For this review, take the finished solid that the model builds, in its own axes (mm). Face numbers are marked on the shaded views. A direction names the side the tool comes from. Round coordinates to 2 decimals unless told otherwise and drop trailing zeros. Order: outer loops, then holes, each group sorted by start corner. A loop starts at its lowest first (then second) coordinate and runs counter-clockwise, first axis right, second up.
from build123d import *

# Parameters (mm, degrees)
SKETCH1_W           = 119.38
SKETCH1_H           = 35.56
BOSS_EXTRUDE1_DEPTH = 37.338
SKETCH2_W           = 10.414
SKETCH2_H           = 31.242
SKETCH2_W_2         = 20.574
CUT_EXTRUDE1_DEPTH  = 117.856
CUT_EXTRUDE2_REACH  = 39.338
SKETCH3_W           = 91.186
SKETCH3_H           = 18.034
SKETCH3_H_2         = 7.874


with BuildPart() as part:
    # Sketch1 → Boss-Extrude1 (new body)
    with BuildSketch(Plane(origin=(0, 0, 0), x_dir=(1, 0, 0), z_dir=(0, 1, 0))):
        Rectangle(SKETCH1_W, SKETCH1_H)
    extrude(amount=BOSS_EXTRUDE1_DEPTH)

    # Sketch2 → Cut-Extrude1 (cut)
    with BuildSketch(Plane(origin=(59.69, 0, 0), x_dir=(0, 0, -1), z_dir=(1, 0, 0))):
        with Locations((-11.049, 18.161)):
            Rectangle(SKETCH2_W, SKETCH2_H)
        with Locations((5.969, 18.161)):
            Rectangle(SKETCH2_W_2, SKETCH2_H)
    extrude(amount=-CUT_EXTRUDE1_DEPTH, mode=Mode.SUBTRACT)

    # Sketch3 → Cut-Extrude2 (cut, up to next)
    with BuildSketch(Plane(origin=(0, 37.338, 0), x_dir=(1, 0, 0), z_dir=(0, 1, 0)), mode=Mode.PRIVATE) as cut_extrude2_sk1:
        with Locations((-11.303, 5.969)):
            Rectangle(SKETCH3_W, SKETCH3_H)
    cut_extrude2_tool1 = extrude(cut_extrude2_sk1.sketch, amount=-CUT_EXTRUDE2_REACH, mode=Mode.PRIVATE) & part.part
    add(cut_extrude2_tool1.solids().sort_by_distance((-11.303, 37.338, -5.969))[0], mode=Mode.SUBTRACT)
    # Sketch3 → Cut-Extrude2 (cut, up to next)
    with BuildSketch(Plane(origin=(0, 37.338, 0), x_dir=(1, 0, 0), z_dir=(0, 1, 0)), mode=Mode.PRIVATE) as cut_extrude2_sk2:
        with Locations((-11.303, -11.049)):
            Rectangle(SKETCH3_W, SKETCH3_H_2)
    cut_extrude2_tool2 = extrude(cut_extrude2_sk2.sketch, amount=-CUT_EXTRUDE2_REACH, mode=Mode.PRIVATE) & part.part
    add(cut_extrude2_tool2.solids().sort_by_distance((-11.303, 37.338, 11.049))[0], mode=Mode.SUBTRACT)


solid = part.part
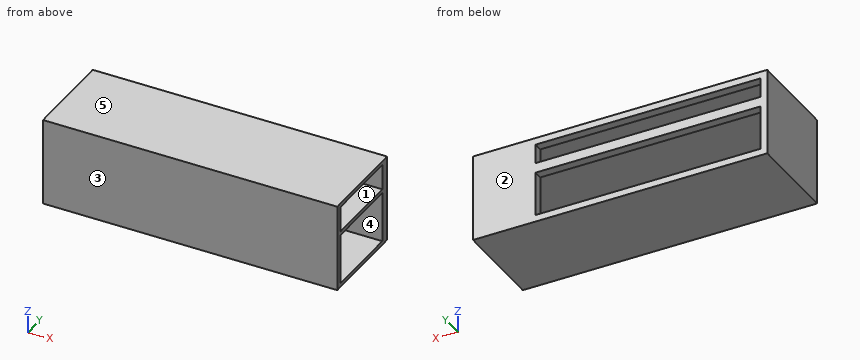
(1) Add section A-A on x = 44. Give the boundary of the cut face in (y, z).
(2) Clearance check with flat-ended pins moving along their axes: P1, Ø2, axis at y = 19, z = 1, coming from the +X side; P2, Ø1, axis at x = -16.5, z = -2.5, coming from the +Y side. State where each tip first meets the part, or that it passes through.
(3) Add section B-B on z = -2.5. Give the boundary of the cut face in (x, y).
(4) Wall thickness on L1, parallel to Z at x = -28, y = 12.5; L2, parallel to Z at x = -17, y = 35; L3, parallel to Y at x = 49.5, z = -9: over which ranges is each line inside the solid? List them lowest first.
(5) Draft analysis for pull direction Y (two halves, no side actions). For the marked faces 3, 4 and 5, state which applies: pulls with the +Y half, pulls with the -Y half, needs draft (parallel to the pull), parting line crosses it, or undercut.
(6) Tool access review of the marked faces 1 and 2: name each direction out of +Z, -Z, +X, -X, +Y, -Y from which nothing blocks a thin tool from reaching the whole face with its end or side.
(7) Add section C-C on y = 21.5. Give the boundary of the cut face in (x, z).
(8) Add section D-D on x = -25.5. Give the boundary of the cut face in (y, z), plus the area to 3 significant figures.
Here are the results:
1. outline: (0, -17.78) - (37.34, -17.78) - (37.34, 17.78) - (0, 17.78) - close; hole (2.54, -16.26) - (33.78, -16.26) - (33.78, 4.32) - (2.54, 4.32) - close; hole (2.54, 5.84) - (33.78, 5.84) - (33.78, 16.26) - (2.54, 16.26) - close
2. P1: stops at x = -58.17
2. P2: stops at y = 2.54
3. outline: (-59.69, 0) - (59.69, 0) - (59.69, 2.54) - (-58.17, 2.54) - (-58.17, 33.78) - (-56.9, 33.78) - (-56.9, 37.34) - (-59.69, 37.34) - close; (34.29, 33.78) - (59.69, 33.78) - (59.69, 37.34) - (34.29, 37.34) - close
4. L1: z = -17.78 to -16.26, 4.32 to 5.84, 16.26 to 17.78
4. L2: z = -17.78 to -14.99, 3.05 to 7.11, 14.99 to 17.78
4. L3: y = 0 to 2.54, 33.78 to 37.34
5. face 3: pulls with the -Y half
5. face 4: undercut
5. face 5: needs draft
6. face 1: +X
6. face 2: +Z, -Z, +X, -X, +Y
7. outline: (-59.69, -17.78) - (59.69, -17.78) - (59.69, -16.26) - (-58.17, -16.26) - (-58.17, 4.32) - (59.69, 4.32) - (59.69, 5.84) - (-58.17, 5.84) - (-58.17, 16.26) - (59.69, 16.26) - (59.69, 17.78) - (-59.69, 17.78) - close
8. outline: (0, -17.78) - (37.34, -17.78) - (37.34, -14.99) - (33.78, -14.99) - (33.78, -16.26) - (2.54, -16.26) - (2.54, 4.32) - (33.78, 4.32) - (33.78, 3.05) - (37.34, 3.05) - (37.34, 7.11) - (33.78, 7.11) - (33.78, 5.84) - (2.54, 5.84) - (2.54, 16.26) - (33.78, 16.26) - (33.78, 14.99) - (37.34, 14.99) - (37.34, 17.78) - (0, 17.78) - close
8. area: 267 mm2
